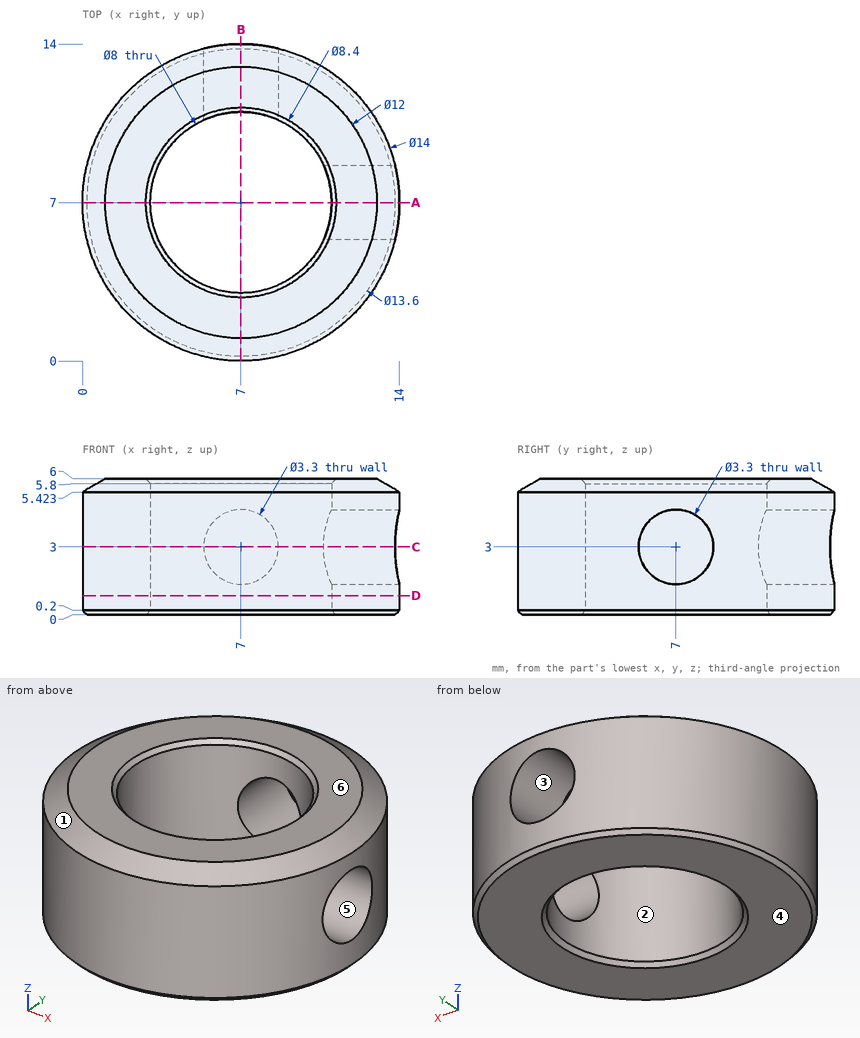
Here's the drawing with two shaded views (mm, measured from the low corner). I have some questions. A direction names the side the tool comes from. Round coordinates to 2 decimals unless told otherwise and drop trailing zeros. Loops run counter-clockwise (first coordinate to the right, second up) from the corner with the lowest first, then second, coordinate; pieces in that order, holes last. Notation, with made-up numbers: (-22.75, 12.5) - (-5.75, 12.5) arc R20 cw to (-5.75, 48.5) - close; hole circle Ø9 at (-15, -17). An arc over 180 degrees is marked (long way). Use CSV: the item, a comma, the result in double quotes. Start each with the question number.
1) Please list where these lines run through material, in increasing order: probe 1 along X at (y, z) = (5, 3.7) (1 decimal); probe 2 along Y at (x, z) = (12.25, 3); probe 3 along Y at (x, z) = (12.75, 1.7) (1 decimal). Write a range as [from, to].
2) If we section it at C-C on z = 3: Write out the boundary of the cut face in (x, y).
3) For the marked faces 5 and 6, which set-ups out of +Z, -Z, +X, -X, +Y, -Y let a thin tool reach every point of the face, with its end or its side?
4) If we section it at D-D on z = 0.85: Write out the boundary of the cut face in (x, y).
5) We'd pull the mould along X, two halves only. Please class the marked faces 1, 2, 3 and 4: released by +X, released by -X, zero draft, split by the parting line, or undercut.
6) For pin 1 Ø2.5 at (x, z) = (7, 3) entering from +Y, with a flat end and sliding along its axis, tell me the tip position at first contact or that it passes through.
7) If we section it at A-A on y = 7: Write out the boundary of the cut face in (x, z), plus the area to 3 significant figures.
Geometry results:
1,probe 1,"x = [0.3, 3.5], [10.5, 13.7]"
1,probe 2,"y = [2.37, 5.35], [8.65, 11.63]"
1,probe 3,"y = [3, 6], [8, 11]"
2,outline,"(5.35, 10.64) - (5.35, 13.8) arc R7 ccw (long way) to (13.8, 5.35) - (10.64, 5.35) arc R4 cw (long way) to start; (8.65, 10.64) arc R4 cw to (10.64, 8.65) - (13.8, 8.65) arc R7 ccw to (8.65, 13.8) - close"
3,face 5,"+X"
3,face 6,"+Z, +X, -X, +Y, -Y"
4,outline,"circle Ø14 at (7, 7); hole circle Ø8 at (7, 7)"
5,face 1,"split by the parting line"
5,face 2,"undercut"
5,face 3,"undercut"
5,face 4,"zero draft"
6,pin 1,"stops at y = 3.2"
7,outline,"(0, 0.2) - (0.2, 0) - (2.8, 0) - (3, 0.2) - (3, 5.8) - (2.8, 6) - (1, 6) - (0, 5.42) - close; (11, 0.2) - (11.2, 0) - (13.8, 0) - (14, 0.2) - (14, 1.35) - (11, 1.35) - close; (11, 4.65) - (14, 4.65) - (14, 5.42) - (13, 6) - (11.2, 6) - (11, 5.8) - close"
7,area,"25.4 mm2"
